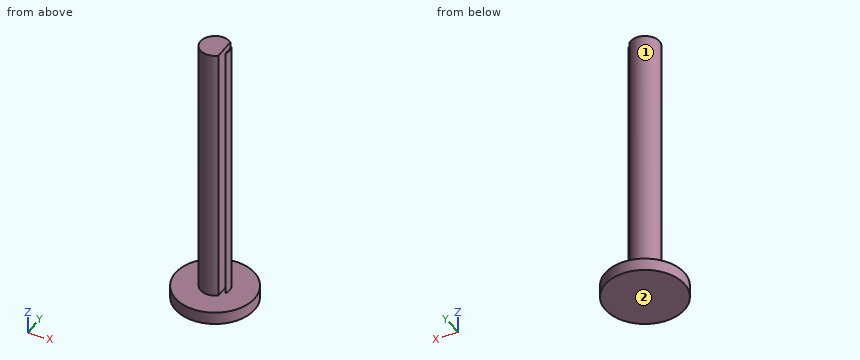
from build123d import *

# Parameters (mm, degrees)
F0_R     = 9.525
F1_DEPTH = 3
F2_R     = 3.5
F3_DEPTH = 63.5
F4_W     = 0.965913
F4_H     = 11.590985
F5_DEPTH = 63.5


with BuildPart() as f1:
    # F0 (on Top) → F1 (new body)
    with BuildSketch(Plane.XY):
        Circle(F0_R)
    extrude(amount=F1_DEPTH)

    # F2 (on face) → F3 (join)
    with BuildSketch(Plane.XY.offset(3)):
        Circle(F2_R)
    extrude(amount=F3_DEPTH)

    # F4 (on face) → F5 (cut)
    with BuildSketch(Plane.XY.offset(66.5)):
        with Locations((2.736762, -0.194345)):
            Rectangle(F4_W, F4_H)
    extrude(amount=-F5_DEPTH, mode=Mode.SUBTRACT)


solid = f1.part
The listing builds one solid part. Answer for the finished solid, in the listing's coordinates (mm). Face numbers are marked on the shaded views. A direction names the side the tool comes from. Give positions to 0.01 mm unless a question says otherwise; leave off trailing zeros. Loops run counter-clockwise (first coordinate to the right, second up) from the corner with the lowest first, then second, coordinate; pieces in that order, holes last.
Item 1: A cutting plane is placed at D-D (y = -6.75). Give the vertices of the cut face in (x, z).
Derived:
outline: (-6.72, 0) - (6.72, 0) - (6.72, 3) - (-6.72, 3) - close
Item 2: Each of these flat-tipped pins is pushed along its axis until it touches: pin 1 Ø1.5 at (x, z) = (5.5, 47) entering from +Y; pin 2 Ø2 at (y, z) = (0, 34) entering from -X; pin 3 Ø3 at (y, z) = (3, 20) entering from +X; pin 4 Ø4 at (x, z) = (0.5, 35.5) entering from -Y. Where does it stop, or does it pass through?
Derived:
pin 1: passes through
pin 2: stops at x = -3.5
pin 3: stops at x = 2.25
pin 4: stops at y = -3.5
Item 3: A cutting plane is placed at C-C (z = 56). Give the vertices of the cut face in (x, y).
Derived:
outline: (2.25, -2.68) - (2.25, 2.68) arc R3.5 ccw (long way) to start; (3.22, -1.37) arc R3.5 ccw to (3.22, 1.37) - close
Item 4: A cutting plane is placed at A-A (x = 0). Give the vertices of the cut face in (y, z) (3 decimals).
Derived:
outline: (-9.525, 0) - (9.525, 0) - (9.525, 3) - (3.5, 3) - (3.5, 66.5) - (-3.5, 66.5) - (-3.5, 3) - (-9.525, 3) - close
Item 5: Find the intervals of material crossed by line 1 along Z through (x, y) = (-2, -3); line 2 along Y through (x, z) = (0, 55); line 3 along X through (y, z) = (2.25, 24.5), in increasing order.
Derived:
line 1: z = 0 to 3
line 2: y = -3.5 to 3.5
line 3: x = -2.68 to 2.25
Item 6: A tool of negligible diameter and unlimited length cuts with its end or side. For the marked faces 1 and 2, from which of +Z, -Z, +X, -X, +Y, -Y can it reach the whole face along a straight path? Write none if from no direction.
Derived:
face 1: +Z
face 2: -Z, +X, -X, +Y, -Y
Item 7: A cutting plane is placed at B-B (y = 0). Give the vertices of the cut face in (x, z) (3 decimals), then the cut area to 3 significant figures.
Derived:
outline: (-9.525, 0) - (9.525, 0) - (9.525, 3) - (3.5, 3) - (3.5, 66.5) - (3.22, 66.5) - (3.22, 3) - (2.254, 3) - (2.254, 66.5) - (-3.5, 66.5) - (-3.5, 3) - (-9.525, 3) - close
area: 440 mm2
